Autodesk Fusion 360 part; units mm, degrees
sketch "スケッチ1" plane through (0, 0, 0) normal (0, 0, 1) x (1, 0, 0)
  line L0 (-40.0294, 0) -> (-27.2294, 0)
  line L1 (-27.2294, 0) -> (-27.2294, -2.8335)
  line L2 (-27.2294, -2.8335) -> (-40.0294, -2.8335)
  line L3 (-40.0294, -2.8335) -> (-40.0294, 0)
  line L4 (-40.0294, 0) -> (-39.0294, 0)
  line L5 (-39.0294, 0) -> (-39.0294, 39.9696)
  line L6 (-39.0294, 39.9696) -> (-40.0294, 39.9696)
  line L7 (-40.0294, 39.9696) -> (-40.0294, 0)
  line L8 (-27.2294, 0) -> (-28.3294, 0)
  line L9 (-28.3294, 0) -> (-28.3294, 40)
  line L10 (-28.3294, 40) -> (-27.2294, 40)
  line L11 (-27.2294, 40) -> (-27.2294, 0)
  line L12 (-27.2294, 0) -> (2.7706, 0)
  line L13 (2.7706, 0) -> (2.7706, -2.9213)
  line L14 (2.7706, -2.9213) -> (-27.2294, -2.9213)
  line L15 (-27.2294, -2.9213) -> (-27.2294, 0)
  line L16 (-12.2294, 0) -> (-12.2294, -2.9213)
  line L17 (2.7706, 0) -> (2.7706, -2.8335)
  line L18 (15.5706, 0) -> (2.7706, 0)
  line L19 (15.5706, 39.9696) -> (15.5706, 0)
  line L20 (3.8706, 0) -> (3.8706, 40)
  line L21 (14.5706, 39.9696) -> (15.5706, 39.9696)
  line L22 (15.5706, 0) -> (14.5706, 0)
  line L23 (14.5706, 0) -> (14.5706, 39.9696)
  line L24 (15.5706, -2.8335) -> (15.5706, 0)
  line L25 (2.7706, -2.9213) -> (2.7706, 0)
  line L26 (2.7706, 40) -> (2.7706, 0)
  line L27 (2.7706, 0) -> (3.8706, 0)
  line L28 (3.8706, 40) -> (2.7706, 40)
  line L29 (2.7706, -2.8335) -> (15.5706, -2.8335)
  line L30 (-27.2294, 40) -> (-25, 35)
  line L31 (-25, 35) -> (-27.2294, 35)
  line L32 (3.8706, 40) -> (2.7706, 40)
  line L33 (0.5411, 35) -> (2.7706, 35)
  line L34 (2.7706, 40) -> (0.5411, 35)
  dimension "d1" = 12.8
  dimension "d2" = 1
  dimension "d3" = 1.1
  dimension "d4" = 30
sketch "スケッチ2" plane through (0, 0, 0) normal (0, 0, 1) x (1, 0, 0)
  line L0 (-40, 34.6932) -> (-40, 33.4932)
  line L1 (-40, 33.4932) -> (-41.2402, 33.4932)
  line L2 (-41.2402, 33.4932) -> (-41.2402, 30.9431)
  line L3 (-41.2402, 30.9431) -> (-40, 30.9431)
  line L4 (-40, 30.9431) -> (-40, 33.4932)
  line L5 (-26, 34.6932) -> (-26, 33.4932)
  line L6 (-27.2402, 33.4932) -> (-27.2402, 30.9431)
  line L7 (-26, 30.9431) -> (-26, 33.4932)
  line L8 (-26, 33.4932) -> (-27.2402, 33.4932)
  line L9 (-27.2402, 30.9431) -> (-26, 30.9431)
  line L10 (-40, 33.4932) -> (-41.2402, 33.4932)
  line L11 (-40, 30.9431) -> (-40, 33.4932)
  line L12 (-41.2402, 33.4932) -> (-41.2402, 30.9431)
  line L13 (-41.2402, 30.9431) -> (-40, 30.9431)
  line L14 (-27.2402, 33.4932) -> (-27.2402, 30.9431)
  line L15 (-26, 33.4932) -> (-27.2402, 33.4932)
  line L16 (-27.2402, 30.9431) -> (-26, 30.9431)
  line L17 (-26, 34.6932) -> (-26, 33.4932)
  line L18 (-26, 30.9431) -> (-26, 33.4932)
  line L19 (-40, 34.6932) -> (-40, 33.4932)
  line L20 (-12.2294, 0) -> (-12.2294, -2.9213)
  line L21 (2.7813, 33.4932) -> (2.7813, 30.9431)
  line L22 (15.5411, 30.9431) -> (15.5411, 33.4932)
  line L23 (16.7813, 33.4932) -> (16.7813, 30.9431)
  line L24 (1.5411, 34.6932) -> (1.5411, 33.4932)
  line L25 (1.5411, 30.9431) -> (1.5411, 33.4932)
  line L26 (2.7813, 33.4932) -> (2.7813, 30.9431)
  line L27 (15.5411, 33.4932) -> (16.7813, 33.4932)
  line L28 (1.5411, 34.6932) -> (1.5411, 33.4932)
  line L29 (2.7813, 30.9431) -> (1.5411, 30.9431)
  line L30 (2.7813, 30.9431) -> (1.5411, 30.9431)
  line L31 (1.5411, 33.4932) -> (2.7813, 33.4932)
  line L32 (1.5411, 33.4932) -> (2.7813, 33.4932)
  line L33 (15.5411, 34.6932) -> (15.5411, 33.4932)
  line L34 (15.5411, 33.4932) -> (16.7813, 33.4932)
  line L35 (16.7813, 33.4932) -> (16.7813, 30.9431)
  line L36 (16.7813, 30.9431) -> (15.5411, 30.9431)
  line L37 (16.7813, 30.9431) -> (15.5411, 30.9431)
  line L38 (1.5411, 30.9431) -> (1.5411, 33.4932)
  line L39 (15.5411, 34.6932) -> (15.5411, 33.4932)
  line L40 (15.5411, 30.9431) -> (15.5411, 33.4932)
  dimension "d8" = 1.2
  dimension "d9" = 1.2
  dimension "d10" = 1.2
  dimension "d11" = 1.2
extrude "押し出し1" add sketch "スケッチ1" sketch "スケッチ2" along normal blind 25.8 of sketch 2
move_face "面をオフセット1" offset 1.5 1 faces at (-28.3294, 26.6667, 17.2)
move_face "面をオフセット2" offset 1.5 1 faces at (3.8706, 26.6667, 17.2)
sketch "スケッチ3" plane through (0, 0, 0) normal (0, 0, 1) x (1, 0, 0)
  line L0 (-22.2393, 22.0314) -> (-2.2393, 22.0314)
  line L1 (-2.2393, 22.0314) -> (-2.2393, 2.0314)
  line L2 (-2.2393, 2.0314) -> (-22.2393, 2.0314)
  line L3 (-22.2393, 2.0314) -> (-22.2393, 22.0314)
  line L4 (-29, 25) -> (4, 25)
  line L5 (4, 25) -> (4, -2)
  line L6 (4, -2) -> (-29, -2)
  line L7 (-29, -2) -> (-29, 25)
  dimension "d16" = 20
  dimension "d17" = 20
extrude "押し出し2" add sketch "スケッチ3" along normal blind 3
sketch "スケッチ4" plane through (0, 0, 0) normal (0, 0, 1) x (1, 0, 0)
  line L0 (-12, -2) -> (-67, -2)
  line L1 (-67, -2) -> (-67, -4)
  line L2 (-67, -4) -> (-12, -4)
  line L3 (-12, -4) -> (-12, -2)
  line L4 (-67, -2) -> (-65, -4)
  line L5 (-65, -4) -> (-85, -24)
  line L6 (-85, -24) -> (-87, -22)
  line L7 (-87, -22) -> (-67, -2)
  line L8 (61, -24) -> (63, -22)
  line L9 (41, -4) -> (61, -24)
  line L10 (-12, -2) -> (43, -2)
  line L11 (43, -2) -> (41, -4)
  line L12 (63, -22) -> (43, -2)
  line L13 (43, -2) -> (43, -4)
  line L14 (43, -4) -> (-12, -4)
  point P0 (-24, 0)
extrude "押し出し3" add sketch "スケッチ4" along normal blind 30
move_face "面をオフセット3" offset 1 1 faces at (33.8569, -2, 18.6)
Could you check a few things on this model? Use its own coordinates, in mm. A direction names the side the tool comes from. Coordinates: 2 decimals unless noted, no trailing zeros. Loops run counter-clockwise (first coordinate to the right, second up) from the corner with the lowest first, then second, coordinate; pieces in that order, holes last. Notation, with made-up numbers: M 85.25,57.25 L 118.25,57.25 A20 cw 118.25,67.25 Z; hole C 3.25,9.5 d8. An arc over 180 degrees is marked long. Put each result on its own line as item: value. Start each with the question number.
(1) Suppose I cut it at B-B on x = -6.5. Please give me the cut outline in (y, z), then the cut area to 3 significant figures.
(2) Suppose I cut it at A-A on y = 10. Please give me the cut outline in (x, z).
(3) Will these pins go through, and if not, where does the flat tip stop? P1, Ø10, axis at x = -11, y = 29, coming from the +Z side; P2, Ø1, axis at x = -38, z = 7, coming from the -Y side; P3, Ø3, axis at y = 35.5, z = 10, coming from the +X side; P4, Ø4, axis at x = -43.5, y = 20, coming from the +Z side.
(4) Suppose I cut it at D-D on x = -33.5. Please give me the cut outline in (y, z).
(5) I need wall thicknesses on line 1 (X direction, y = 9, z = 16.5); line 2 (X direction, y = 12, z = 2); line 3 (Y direction, x = 13, z = 12). Which ranges of each line are inside material? Lowest first, please. Write a range as from..to.
(6) Thinking about a two-plate mould opening in X: for faces 4 (the face through (16.781, 32, 13)), 5 (the face through (-7, 1, 0)), 6 (the face through (5.371, 20, 13)), which applies, pulls with the +X half, pulls with the -X half, needs draft (parallel to the pull), parting line crosses it, or undercut?
(7) For faces 1 (the face through (-26, 32, 13)), 2 (the face through (2.771, 16, 13)), 3 (the face through (10, 0, 13)), which set-ups out of +Z, -Z, +X, -X, +Y, -Y let a thin tool reach every point of the face, with its end or its side?
(8) Suppose I cut it at C-C on y = -13. Please give me the cut outline in (x, z), then the cut area to 3 significant figures.
Solutions:
1. outline: M -4,0 L 2.03,0 L 2.03,3 L 0,3 L 0,25.8 L -1,25.8 L -1,30 L -4,30 Z; M 22.03,0 L 25,0 L 25,3 L 22.03,3 Z
1. area: 131 mm2
2. outline: M -40.03,0 L -39.03,0 L -39.03,25.8 L -40.03,25.8 Z; M -29.83,0 L -22.24,0 L -22.24,3 L -27.23,3 L -27.23,25.8 L -29.83,25.8 Z; M -2.24,0 L 5.37,0 L 5.37,25.8 L 2.77,25.8 L 2.77,3 L -2.24,3 Z; M 14.57,0 L 15.57,0 L 15.57,25.8 L 14.57,25.8 Z
3. P1: stops at z = 3
3. P2: stops at y = -4
3. P3: stops at x = 15.57
3. P4: passes through
4. outline: M -4,0 L 0,0 L 0,25.8 L -1,25.8 L -1,30 L -4,30 Z
5. line 1: x = -40.03..-39.03, -29.83..-27.23, 2.77..5.37, 14.57..15.57
5. line 2: x = -40.03..-39.03, -29.83..-22.24, -2.24..5.37, 14.57..15.57
5. line 3: y = -4..0
6. face 4: pulls with the +X half
6. face 5: needs draft
6. face 6: undercut
7. face 1: +Z, -Z
7. face 2: +Z
7. face 3: +Z, -Z, +Y
8. outline: M -78,0 L -74,0 L -74,30 L -78,30 Z; M 50,0 L 54,0 L 54,30 L 50,30 Z
8. area: 240 mm2
